The listing builds one solid part. Answer for the finished solid, in the listing's coordinates (mm). Face numbers are marked on the shaded views. A direction names the side the tool comes from. Give positions to 0.01 mm unless a question says otherwise; leave off trailing zeros. Order: outer loops, then holes, each group sorted by start corner. A loop starts at its lowest first (then second) coordinate and runs counter-clockwise, first axis right, second up. Notation, with made-up numbers: (81, 63.25) - (112, 63.25) arc R33 cw to (112, 102.25) - close; hole circle Ø3 at (81, 0.25). An arc over 180 degrees is marked (long way). Answer as a JSON object with one key per item and string values. Group by question number.
Q1. A cutting plane is placed at D-D, the plane x = 4.75. Count the separate pieces of the cut face and the enclosed holes in it, and give its area (3 significant figures).
Q2. A cutting plane is placed at B-B, the plane y = 26. Give the vertices of the cut face in (x, z).
Q3. A cutting plane is placed at C-C, the plane z = 0. Give the vertices of the cut face in (x, y), and give its area (3 significant figures).
Q4. A cutting plane is placed at A-A, the plane y = 13. Give the vertices of the cut face in (x, z), and give its area (3 significant figures).
Q5. For the marked faces 4, 5 and 6, determine the directions among +Z, -Z, +X, -X, +Y, -Y from which every point of the face is accessible in a straight line to the end or side of a thin tool.
Q6. Consider line 1 (Z direction, x = 2.25, y = 28); line 2 (Y direction, x = 10.75, z = 13); line 3 (Z direction, x = 7, y = -6.5). Determine where each line is inside the solid, lowest interval first.
Q7. The mould has two halves that part along Z. Classify the marked faces 1, 2 and 3: released by +Z, released by -Z, zero draft, split by the parting line, or undercut.
Q8. Given pin 1 (1 mm diameter, centred on x = 12, z = -9.5, fed in from +Y); pin 2 (6 mm diameter, centred on x = 5.5, z = -5.5, fed in from -Y); pin 3 (4 mm diameter, centred on x = 5, z = -12, fed in from +Y), each flat-ended and moving along its own axis, determine where each tip first touches the part or whether it passes through.
from build123d import *

# Parameters (mm, degrees)
F1_DEPTH      = 10
F1_DEPTH_BACK = 10
F5_DEPTH      = 28
F8_D          = 23.62
F9_D          = 2.8
F9_ON_F2_D    = 2.8
F10_D         = 3.4
F10_ON_F2_D   = 3.4
F7_W          = 14
F7_H          = 23.5
F11_DEPTH     = 25
F12_T1_DEPTH  = 30


# Not quite as in the source:
# - a fillet or chamfer that OpenCascade refuses, or shapes differently, is made with other operations: its cross-section is extruded or revolved along the edge and cut away or added


with BuildPart() as f1:
    # F0 (on Front) → F1 (new body, two sides)
    with BuildSketch(Plane.XZ) as f1_sk:
        with BuildLine():
            Line((15, 17), (0, 17))
            Line((0, 17), (0, 11.81))
            ThreePointArc((0, 11.81), (8.3509310858, 8.3509310858), (11.81, 0))
            ThreePointArc((11.81, 0), (8.3509310858, -8.3509310858), (0, -11.81))
            Line((0, -11.81), (0, -17))
            Line((0, -17), (15, -17))
            Line((15, -17), (15, 17))
        make_face()
    extrude(amount=F1_DEPTH)
    extrude(f1_sk.sketch, amount=-F1_DEPTH_BACK)

    # F2 (on face) → F3 (revolve, cut)
    with BuildSketch(Plane(origin=(0, 0, 0), x_dir=(0, -1, 0), z_dir=(-1, 0, 0))):
        with BuildLine():
            Line((-1.25, -11.81), (1.25, -11.81))
            ThreePointArc((1.25, -11.81), (0, -10.56), (-1.25, -11.81))
        make_face()
        with BuildLine():
            ThreePointArc((-1.25, -11.81), (0, -13.06), (1.25, -11.81))
            Line((1.25, -11.81), (-1.25, -11.81))
        make_face()
    revolve(axis=Axis((0, 0, 0), (0, -1, 0)), mode=Mode.SUBTRACT)

    # F4 (on face) → F5 (join)
    with BuildSketch(Plane(origin=(0, 10, 0), x_dir=(-1, 0, 0), z_dir=(0, 1, 0))):
        with BuildLine():
            Line((0, -11.81), (0, 11.81))
            ThreePointArc((0, 11.81), (-11.81, 0), (0, -11.81))
        make_face()
        with BuildLine():
            Line((0, 17), (-15, 17))
            Line((-15, 17), (-15, -17))
            Line((-15, -17), (0, -17))
            Line((0, -17), (0, -11.81))
            ThreePointArc((0, -11.81), (-11.81, 0), (0, 11.81))
            Line((0, 11.81), (0, 17))
        make_face()
    extrude(amount=F5_DEPTH)

    # F6: union 

    # F8 (through all)
    with Locations(Plane(origin=(0, 0, 0), x_dir=(0, -1, 0), z_dir=(-1, 0, 0))):
        with Locations((-24, 0)):
            Hole(F8_D / 2)

    # F9 (through all)
    with Locations(Plane(origin=(0, 0, 0), x_dir=(0, -1, 0), z_dir=(-1, 0, 0))):
        with Locations((-13.5, 14)):
            Hole(F9_D / 2)

    # F9 on F2 (through all)
    with Locations(Plane(origin=(0, 0, 0), x_dir=(0, -1, 0), z_dir=(-1, 0, 0))):
        with Locations((6.5, -14)):
            Hole(F9_ON_F2_D / 2)

    # F10 (through all)
    with Locations(Plane(origin=(0, 0, 0), x_dir=(0, -1, 0), z_dir=(-1, 0, 0))):
        with Locations((-13.5, -14)):
            Hole(F10_D / 2)

    # F10 on F2 (through all)
    with Locations(Plane(origin=(0, 0, 0), x_dir=(0, -1, 0), z_dir=(-1, 0, 0))):
        with Locations((6.5, 14)):
            Hole(F10_ON_F2_D / 2)

    # F7 (on face) → F11 (cut)
    with BuildSketch(Plane(origin=(0, 0, 0), x_dir=(0, -1, 0), z_dir=(-1, 0, 0))):
        with Locations((-31, 0)):
            Rectangle(F7_W, F7_H)
    extrude(amount=-F11_DEPTH, mode=Mode.SUBTRACT)

    # F12: fillet of radius 3 on 6 edges, made by hand

    # F12_s2 → F12_t1 (cut)
    with BuildSketch(Plane.YZ.offset(-7.5)):
        with BuildLine():
            ThreePointArc((-7, -17), (-9.1213203436, -16.1213203436), (-10, -14))
            Line((-10, -14), (-10, -17))
            Line((-10, -17), (-7, -17))
        make_face()
        with BuildLine():
            ThreePointArc((-7, 17), (-9.1213203436, 16.1213203436), (-10, 14))
            Line((-10, 14), (-10, 17))
            Line((-10, 17), (-7, 17))
        make_face()
        with BuildLine():
            ThreePointArc((38, -14), (37.1213203436, -16.1213203436), (35, -17))
            Line((35, -17), (38, -17))
            Line((38, -17), (38, -14))
        make_face()
        with BuildLine():
            ThreePointArc((35, 17), (37.1213203436, 16.1213203436), (38, 14))
            Line((38, 14), (38, 17))
            Line((38, 17), (35, 17))
        make_face()
        with BuildLine():
            ThreePointArc((35, -11.75), (37.1213203436, -12.6286796564), (38, -14.75))
            Line((38, -14.75), (38, -11.75))
            Line((38, -11.75), (35, -11.75))
        make_face()
        with BuildLine():
            ThreePointArc((38, 14.75), (37.1213203436, 12.6286796564), (35, 11.75))
            Line((35, 11.75), (38, 11.75))
            Line((38, 11.75), (38, 14.75))
        make_face()
    extrude(amount=F12_T1_DEPTH, mode=Mode.SUBTRACT)


solid = f1.part
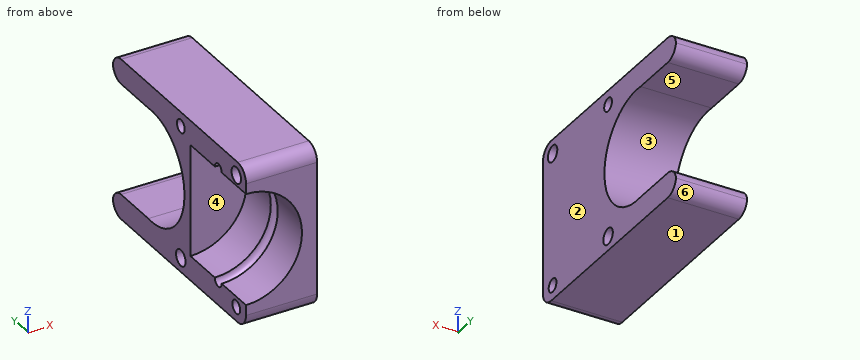
Reply:
{
 "1": {"separate pieces": "1", "enclosed holes": "4", "area": "604 mm^2"},
 "2": {"outline": "(0, -17) - (15, -17) - (15, -11.75) - (0, -11.75) - close; (0, 11.75) - (15, 11.75) - (15, 17) - (0, 17) - close"},
 "3": {"outline": "(0, 10) - (11.81, 10) - (11.81, 1.25) arc R1.25 cw to (11.81, -1.25) - (11.81, -10) - (15, -10) - (15, 12.19) - (0, 12.19) - close", "area": "94.2 mm^2"},
 "4": {"outline": "(0, -17) - (15, -17) - (15, -15.62) - (0, -15.62) - close; (0, -12.38) - (15, -12.38) - (15, -4.3) - (0, -4.3) - close; (0, 4.3) - (15, 4.3) - (15, 12.69) - (0, 12.69) - close; (0, 15.31) - (15, 15.31) - (15, 17) - (0, 17) - close", "area": "293 mm^2"},
 "5": {"face 4": "-X, -Y", "face 5": "+X, -X, +Y", "face 6": "-Z, +X, -X, +Y"},
 "6": {"line 1": "z = -17 to -11.75, 11.75 to 17", "line 2": "y = -10 to -7.87, -5.13 to 12.52, 14.48 to 37.44", "line 3": "z = -17 to -15.4, -12.6 to -9.51, 9.51 to 12.3, 15.7 to 17"},
 "7": {"face 1": "released by -Z", "face 2": "zero draft", "face 3": "undercut"},
 "8": {"pin 1": "stops at y = 17.72", "pin 2": "stops at y = 10", "pin 3": "stops at y = 37.9"}
}
